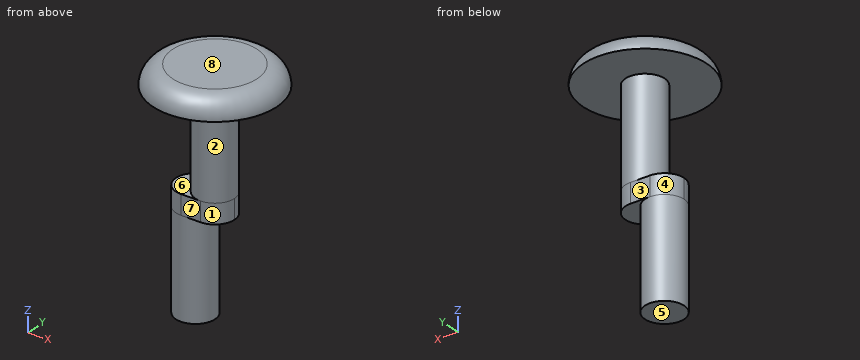
from build123d import *

# Parameters (mm, degrees)
F0_R     = 5
F1_DEPTH = 25
F2_W     = 15
F2_H     = 10
F3_DEPTH = 5
F4_R     = 5
F5_DEPTH = 25
F6_R     = 4.9999
F7_R     = 15.7954316655
F8_DEPTH = 5
F9_R     = 4.99999


# Not quite as in the source:
# - a fillet or chamfer is up to 0.001 mm smaller than in the source, because OpenCascade refuses the exact size


with BuildPart() as f1:
    # F0 (on Top) → F1 (new body)
    with BuildSketch(Plane.XY):
        Circle(F0_R)
    extrude(amount=F1_DEPTH)

    # F2 (on face) → F3 (join)
    with BuildSketch(Plane.XY.offset(25)):
        with Locations((2.5, 0)):
            Rectangle(F2_W, F2_H)
    extrude(amount=F3_DEPTH)

    # F4 (on face) → F5 (join)
    with BuildSketch(Plane.XY.offset(30)):
        with Locations((5, 0)):
            Circle(F4_R)
    extrude(amount=F5_DEPTH)

    # F6 (radius 5 in the source; OpenCascade refuses exactly that, so slightly less here)
    f6_edges = [f1.edges().sort_by_distance(p)[0] for p in [
        (10, -5, 27.5),
        (10, 5, 27.5),
        (-5, 5, 27.5),
        (-5, -5, 27.5),
    ]]
    fillet(f6_edges, radius=F6_R)

    # F7 (on face) → F8 (join)
    with BuildSketch(Plane.XY.offset(55)):
        with Locations((5, 0)):
            Circle(F7_R)
    extrude(amount=F8_DEPTH)

    # F9 (radius 5 in the source; OpenCascade refuses exactly that, so slightly less here)
    f9_edges = [f1.edges().sort_by_distance(p)[0] for p in [
        (-10.795432, 0, 60),
    ]]
    fillet(f9_edges, radius=F9_R)


solid = f1.part
Here's how the part is built. I have some questions about the finished solid (model axes, mm). Face numbers are marked on the shaded views. A direction names the side the tool comes from. Round coordinates to 2 decimals unless told otherwise and drop trailing zeros. Order: outer loops, then holes, each group sorted by start corner. A loop starts at its lowest first (then second) coordinate and runs counter-clockwise, first axis right, second up. Notation, with made-up numbers: M 70,-11.5 L 119,-11.5 A4 cw 119,-6.5 Z; hole C 17.25,42.5 d3. An arc over 180 degrees is marked long. One line per question, with ' | ' between items.
1) I need wall thicknesses on line 1 (Z direction, x = -5, y = 1.5); line 2 (Y direction, x = 5, z = 45); line 3 (Z direction, x = 1, y = -4). Which ranges of each line are inside material? Lowest first, please.
Checked values:
line 1: z = 55 to 60 | line 2: y = -5 to 5 | line 3: z = 0 to 30, 55 to 60
2) I'm going to push flat-ended pins straight in: pin 1 Ø1.5 at (x, z) = (3.5, 27.5) entering from +Y; pin 2 Ø1.5 at (x, z) = (1.5, 28) entering from -Y; pin 3 Ø6 at (y, z) = (2, 50.5) entering from +X. Where does each tip first touch, or does it pass through?
Checked values:
pin 1: stops at y = 5 | pin 2: stops at y = -5 | pin 3: stops at x = 10
3) On a 3-axis mill with a long thin cutter (end or side, diameter ignored), from which of +Z, -Z, +X, -X, +Y, -Y can I reach the whole of each face in a straight line? I mean the marked faces 1, 2, 3 and 4. Say none if no direction works.
Checked values:
face 1: -Z, +X, -Y | face 2: none | face 3: -Z, +X, -X, +Y | face 4: -Z, -X, +Y
4) We'd pull the mould along Z, two halves only. Please class the marked faces 5, 6, 7 and 8: released by +Z, released by -Z, zero draft, split by the parting line, or undercut.
Checked values:
face 5: released by -Z | face 6: undercut | face 7: zero draft | face 8: released by +Z
5) Imagine slicing it at A-A, the plane z = 56.5. Write out the boundary of the cut face in (x, y), plus the area to 3 significant figures.
Checked values:
outline: C 5,0 d31.13 | area: 761 mm²
